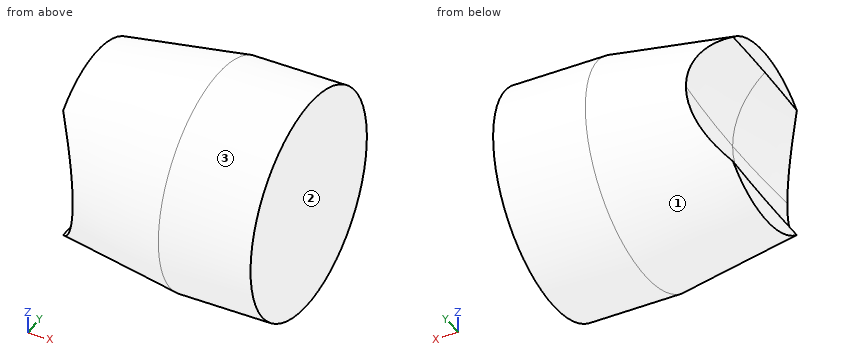
from build123d import *

# Parameters (mm, degrees)
SKETCH001_R = 3.05


with BuildPart() as part:
    # Sketch → Revolution (revolve)
    with BuildSketch(Plane.XZ):
        Polygon((0, 0), (0, 3), (3.95, 3.6), (6.95, 3.6), (6.95, 0), align=None)
    revolve(axis=Axis((0, 0, 0), (1, 0, 0)))

    # Sketch001 → Groove (revolve, cut)
    with BuildSketch(Plane.XZ):
        with Locations((-2, 0)):
            Circle(SKETCH001_R)
    revolve(axis=Axis((-37, 0, 0), (0, 0, 1)), mode=Mode.SUBTRACT)


solid = part.part
Can you work these out from the model? Positions are in its coordinate system, mm. Face numbers are marked on the shaded views. Coordinates: 2 decimals unless noted, no trailing zeros. Write each loop counter-clockwise with the first axis right and the second up, starting at its lowest first coordinate (ties: lowest second). Pieces come first, ordered by that corner, then holes. Notation, with made-up numbers: (54.25, 53.25) -> (65.25, 53.25) arc R25 cw to (65.25, 76.25) -> close; hole circle Ø5 at (78.25, -24). An arc over 180 degrees is marked (long way). Write each question's results on one line, items separated by ' | '. Start each with the question number.
Item 1: Please list where these lines run through material, in increasing order: probe 1 along Z at (x, y) = (5.75, 3.25); probe 2 along Z at (x, y) = (1.75, 1); probe 3 along X at (y, z) = (1, -2.25).
Item 2: If we section it at A-A, the plane x = 6.75: Write out the boundary of the cut face in (y, z).
Item 3: I'm going to push flat-ended pins straight in: P1, Ø1.5, axis at x = 4, y = 1.5, coming from the -Z side; P2, Ø4, axis at x = 3.5, y = 3, coming from the -Z side; P3, Ø1.5, axis at y = -0.5, z = 0, coming from the -X side. Where does each tip first touch, or does it pass through?
Item 4: If we section it at B-B, the plane x = 3.5: Write out the boundary of the cut face in (y, z), and give its area (3 significant figures).
Item 5: Thinking about a two-plate mould opening in X: for the marked faces 1, 2 and 3, which applies, released by +X, released by -X, zero draft, split by the parting line, or undercut?
Answer block:
1) probe 1: -1.55 to 1.55 | probe 2: -3.11 to 3.11 | probe 3: 0.05 to 6.95
2) outline: circle Ø7.2 at (0, 0)
3) P1: z = -3.52 | P2: z = -3.44 | P3: x = 0.95
4) outline: circle Ø7.06 at (0, 0) | area: 39.2 mm²
5) face 1: released by -X | face 2: released by +X | face 3: zero draft
